Can you work these out from the model? Positions are in its coordinate system, mm. Face numbers are marked on the shaded views. A direction names the side the tool comes from. Round coordinates to 2 decimals unless told otherwise and drop trailing zeros. Order: outer loops, then holes, each group sorted by start corner. A loop starts at its lowest first (then second) coordinate and runs counter-clockwise, first axis right, second up. Notation, with made-up numbers: M -27,-8.75 L 7,-8.75 A27 cw 7,18.25 Z; hole C -11.5,-2.75 d9. An arc over 180 degrees is marked long. Answer as a JSON object with one key per item and string values. Group by question number.
```python
from build123d import *

# Parameters (mm, degrees)
F0_W          = 97.1658453345
F0_H          = 57.3885776103
F1_DEPTH      = 44.196
F1_DEPTH_BACK = 44.196
F4_T          = -2.54
F5_START      = 41.656
F2_W          = 96.8622006476
F2_H          = 19.7368133813
F3_W          = 97.1658416092
F3_H          = 16.3967330009
F5_DEPTH      = 2.286


with BuildPart() as f1:
    # F0 (on Top) → F1 (new body, two sides)
    with BuildSketch(Plane.XY) as f1_sk:
        Rectangle(F0_W, F0_H)
    extrude(amount=F1_DEPTH)
    extrude(f1_sk.sketch, amount=-F1_DEPTH_BACK)

    # F4
    f4_openings = [f1.faces().sort_by_distance(p)[0] for p in [
        (0, 0, 44.196),
    ]]
    offset(amount=F4_T, openings=f4_openings)

    # F2 (on Top) + F3 (on Top) → F5 (join)
    with BuildSketch(Plane.XY.offset(F5_START)):
        with Locations((-0.1518223435, 38.5626954958)):
            Rectangle(F2_W, F2_H)
    with BuildSketch(Plane.XY.offset(F5_START)):
        with Locations((-1.8626e-06, -36.8926553056)):
            Rectangle(F3_W, F3_H)
    extrude(amount=F5_DEPTH)


solid = f1.part
```
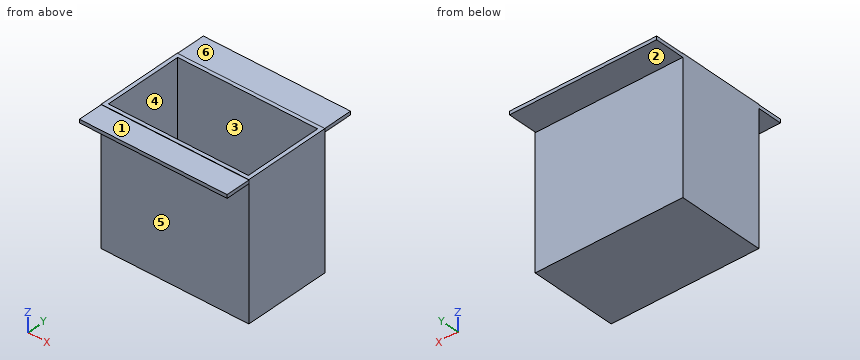
1) If we section it at A-A on z = -24.5: Write out the boundary of the cut face in (x, y).
2) If we section it at C-C on y = -1.5: Write out the boundary of the cut face in (x, z).
3) I need wall thicknesses on line 1 along X through (y, z) = (22, -4); line 2 along Y through (x, z) = (-15, -34); line 3 along Z through (x, y) = (-7, 23). Which ranges of each line are inside material? Lowest first, please.
4) Which directions (+Z, -Z, +X, -X, +Y, -Y) give clear straight access to the entire face, cutting with the end or side of a thin tool? Please do the marked faces 1, 2 and 3.
5) For pin 1 (12 mm diameter, centred on x = -7, y = 35, fed in from +Z); pin 2 (4 mm diameter, centred on x = -23, z = 7, fed in from -Y); pin 3 (8 mm diameter, centred on x = -17, y = -39.5, fed in from -Z), each with a flat end and sliding along its axis, tell me the tip position at first contact or that it passes through.
6) We'd pull the mould along Y, two halves only. Please class the marked faces 4, 5 and 6: +Y half, -Y half, draft (parallel to the pull), parting line (faces both ways), or undercut.
7) If we section it at B-B on x = 25.5: Write out the boundary of the cut face in (y, z), plus the area to 3 significant figures.
8) If we section it at D-D on y = 37: Write out the boundary of the cut face in (x, z).
Findings:
{
 "1": {"outline": "M -48.58,-28.69 L 48.58,-28.69 L 48.58,28.69 L -48.58,28.69 Z; hole M -46.04,-26.15 L 46.04,-26.15 L 46.04,26.15 L -46.04,26.15 Z"},
 "2": {"outline": "M -48.58,-44.2 L 48.58,-44.2 L 48.58,44.2 L 46.04,44.2 L 46.04,-41.66 L -46.04,-41.66 L -46.04,44.2 L -48.58,44.2 Z"},
 "3": {"line 1": "x = -48.58 to -46.04, 46.04 to 48.58", "line 2": "y = -28.69 to -26.15, 26.15 to 28.69", "line 3": "z = -44.2 to -41.66"},
 "4": {"face 1": "+Z, +X, -X, -Y", "face 2": "-Z, +X, -X, +Y", "face 3": "+Z"},
 "5": {"pin 1": "stops at z = 43.94", "pin 2": "stops at y = -28.69", "pin 3": "stops at z = 41.66"},
 "6": {"face 4": "undercut", "face 5": "-Y half", "face 6": "draft"},
 "7": {"outline": "M -45.09,41.66 L -28.69,41.66 L -28.69,-44.2 L 28.69,-44.2 L 28.69,41.66 L 48.43,41.66 L 48.43,43.94 L 28.69,43.94 L 28.69,44.2 L 26.15,44.2 L 26.15,-41.66 L -26.15,-41.66 L -26.15,44.2 L -28.69,44.2 L -28.69,43.94 L -45.09,43.94 Z", "area": "664 mm^2"},
 "8": {"outline": "M -48.58,41.66 L 48.28,41.66 L 48.28,43.94 L -48.58,43.94 Z"}
}
